from build123d import *

# Parameters (mm, degrees)
HOLE1_D           = 4.826
HOLE1_DEPTH       = 26.1874
HOLE1_CSINK_D     = 5.842
HOLE1_CSINK_ANGLE = 90


with BuildPart() as part:
    # Sketch1 → Revolve1 (revolve)
    with BuildSketch(Plane.XY):
        with BuildLine():
            Line((0, 0), (0, 4.8006))
            Line((0, 4.8006), (0.75565, 5.55625))
            Line((0.75565, 5.55625), (4.660293864, 5.55625))
            Line((4.660293864, 5.55625), (5.418103291, 4.804192648))
            ThreePointArc((5.418103291, 4.804192648), (5.676923575, 4.6323221), (5.9817, 4.572))
            Line((5.9817, 4.572), (7.1501, 4.572))
            ThreePointArc((7.1501, 4.572), (7.715856136, 4.806343864), (7.9502, 5.3721))
            Line((7.9502, 5.3721), (7.9502, 5.53085))
            Line((7.9502, 5.53085), (9.525, 5.53085))
            Line((9.525, 5.53085), (9.525, 0))
            Line((9.525, 0), (0, 0))
        make_face()
    revolve(axis=Axis((9.525, 0, 0), (-1, 0, 0)))

    # Sketch2 → Revolve2 (revolve)
    with BuildSketch(Plane.XY):
        Polygon((9.525, 0), (9.525, 7.0485), (10.287, 7.8105), (12.446, 7.8105), (12.7, 7.5565), (12.7, 6.63575), (13.335, 6.63575), (13.97, 7.27075), (18.288, 7.27075), (19.05, 6.50875), (19.05, 0), align=None)
    revolve(axis=Axis((19.05, 0, 0), (-1, 0, 0)))

    # Sketch3 → Revolve3 (revolve)
    with BuildSketch(Plane.XY):
        Polygon((19.05, 0), (19.05, 5.08), (25.4254, 5.08), (26.1874, 4.318), (26.1874, 0), align=None)
    revolve(axis=Axis((26.1874, 0, 0), (-1, 0, 0)))

    # Hole1
    with Locations(Plane.ZY):
        with Locations((0, 0)):
            CounterSinkHole(HOLE1_D / 2, HOLE1_CSINK_D / 2, depth=HOLE1_DEPTH, counter_sink_angle=HOLE1_CSINK_ANGLE)

    # Sketch6 → Revolve4 (revolve)
    with BuildSketch(Plane.XY):
        with BuildLine():
            Line((12.7, 6.38175), (13.335, 6.38175))
            Line((13.335, 6.38175), (13.335, 6.63575))
            Line((13.335, 6.63575), (13.0175, 6.63575))
            Line((13.0175, 6.63575), (12.817039755, 6.836210245))
            ThreePointArc((12.817039755, 6.836210245), (12.779842316, 6.926012806), (12.817039755, 7.015815367))
            Line((12.817039755, 7.015815367), (13.527556192, 7.726331804))
            Line((13.527556192, 7.726331804), (13.527556192, 7.8105))
            Line((13.527556192, 7.8105), (13.324356192, 7.8105))
            Line((13.324356192, 7.8105), (12.7, 7.186143808))
            Line((12.7, 7.186143808), (12.7, 6.38175))
        make_face()
    revolve(axis=Axis((13.335, 0, 0), (-1, 0, 0)))


solid = part.part
The listing builds one solid part. Answer for the finished solid, in the listing's coordinates (mm). A direction names the side the tool comes from. Coordinates: 2 decimals unless noted, no trailing zeros. Loops run counter-clockwise (first coordinate to the right, second up) from the corner with the lowest first, then second, coordinate; pieces in that order, holes last.
1) Find section B-B on x = 7.5. Write down the section's boundary in (y, z).
2) Determine the mould class of faces 4 (the face through (13.527, -1.468, 1.915)), 5 (the face through (9.525, -3, 5)), 6 (the face through (8.749, -4.389, 3.365)), 7 (the face through (13.18, 3.06, 5.89)) for opening direction Y: pulls with the +Y half, pulls with the -Y half, needs draft (parallel to the pull), parting line crosses it, or undercut.
3) Find section A-A on x = 19.75. Write down the section's boundary in (y, z).
4) Find the intervals of material crossed by L1, parallel to Z at x = 11.75, y = 0; L2, parallel to Z at x = 16.5, y = 0; L3, parallel to Y at x = 8.75, z = 0, in increasing order.
5) Flat-ended cylindrical pins translate along their axes: pin 1 Ø8 at (x, z) = (10.5, -4) entering from +Y; pin 2 Ø1 at (x, y) = (4.5, 4.5) entering from +Z; pin 3 Ø2 at (x, z) = (4, -5.5) entering from -Y; pin 4 Ø3 at (x, y) = (3.5, -4.5) entering from -Z. Find the tip coordinate at first contact, or state that the pin passes through.
6) A tool of negligible diameter and unlimited length cuts with its end or side. For faces 1 (the face through (2.74, 5.3, -1.67)), 2 (the face through (0, 0.1, 3.1)), 3 (the face through (22.282, -0.661, -5.037)), from which of +Z, -Z, +X, -X, +Y, -Y can it reach the whole face along a straight path? Write none if from no direction.
Values:
1. outline: circle Ø9.31 at (0, 0); hole circle Ø4.83 at (0, 0)
2. face 4: undercut
2. face 5: needs draft
2. face 6: parting line crosses it
2. face 7: undercut
3. outline: circle Ø10.16 at (0, 0); hole circle Ø4.83 at (0, 0)
4. L1: z = -7.81 to -2.41, 2.41 to 7.81
4. L2: z = -7.27 to -2.41, 2.41 to 7.27
4. L3: y = -5.53 to -2.41, 2.41 to 5.53
5. pin 1: stops at y = 7.81
5. pin 2: stops at z = 3.86
5. pin 3: stops at y = -3.26
5. pin 4: stops at z = -4.68
6. face 1: -X
6. face 2: +Z, -Z, -X, +Y, -Y
6. face 3: +X
